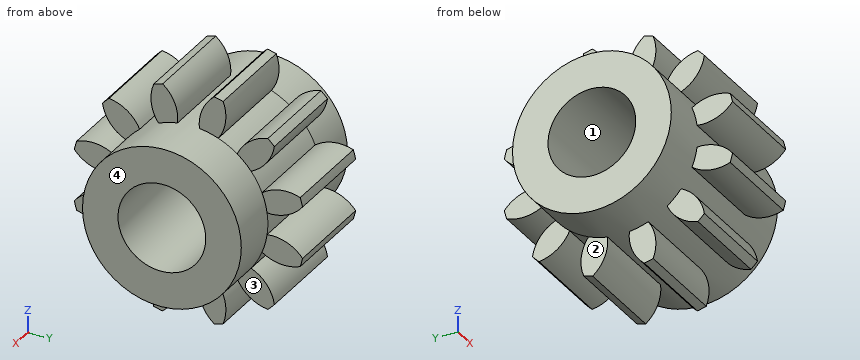
```python
from build123d import *
from build123d.topology import SkipClean

# Parameters (mm, degrees)
BASPROSKE_W       = 25.4
BASPROSKE_H       = 29.633333333
TOOTHCUT_DEPTH    = 50.004376222
TEETHCUTS_COUNT   = 12
TEETHCUTS_ANGLE   = 330
HUBNEABOTSKE_R    = 20.107063333
HUBNEARBOTH_DEPTH = 12.7000254
HUBFARSKE_R       = 20.107063333
HUBFAR_DEPTH      = 12.7000254
BORSKE_R          = 11.1125
BORE_DEPTH        = 50.8000508
SCALE1_SCALE      = 0.39


with BuildPart() as part:
    # BasProSke → Base-Revolve (revolve)
    with BuildSketch(Plane(origin=(0, 0, 0), x_dir=(1, 0, 0), z_dir=(0, 1, 0)), mode=Mode.PRIVATE) as base_revolve_sk:
        with Locations((12.7, 14.816666667)):
            Rectangle(BASPROSKE_W, BASPROSKE_H)
    revolve(base_revolve_sk.sketch.rotate(Axis((-10, 0, 0), (1, 0, 0)), 180), axis=Axis((-10, 0, 0), (1, 0, 0)))

    # TooCutSke → ToothCut (cut, through all)
    with BuildSketch(Plane(origin=(0, 0, 0), x_dir=(0, 0, -1), z_dir=(1, 0, 0))):
        with BuildLine():
            ThreePointArc((2.76285054, 19.91634135), (0, 20.107063333), (-2.76285054, 19.91634135))
            ThreePointArc((-2.76285054, 19.91634135), (-3.510108668, 24.907095847), (-6.566398379, 28.922705186))
            ThreePointArc((-6.566398379, 28.922705186), (0, 29.658733333), (6.566398379, 28.922705186))
            ThreePointArc((6.566398379, 28.922705186), (3.510108668, 24.907095847), (2.76285054, 19.91634135))
        make_face()
    toothcut = extrude(amount=TOOTHCUT_DEPTH, mode=Mode.SUBTRACT)

    # TeethCuts: ToothCut ×12 about axis
    teethcuts_axis = Axis((-10, 0, 0), (1, 0, 0))
    for i in range(1, TEETHCUTS_COUNT):
        add(toothcut.rotate(teethcuts_axis, i * TEETHCUTS_ANGLE / (TEETHCUTS_COUNT - 1)), mode=Mode.SUBTRACT)

    # HubNeaBotSke → HubNearBoth (add)
    with SkipClean():  # the faces are left unmerged after this step: merging them gives an invalid solid
        with BuildSketch(Plane.ZY):
            Circle(HUBNEABOTSKE_R)
        extrude(amount=HUBNEARBOTH_DEPTH)

    # HubFarSke → HubFar (add)
    with SkipClean():  # the faces are left unmerged after this step: merging them gives an invalid solid
        with BuildSketch(Plane(origin=(25.4, 0, 0), x_dir=(0, 0, -1), z_dir=(1, 0, 0))):
            with Locations(Location((0, 0, 0), (0, 0, 180))):
                Circle(HUBFARSKE_R)
        extrude(amount=HUBFAR_DEPTH)

    # BorSke → Bore (cut, symmetric)
    with SkipClean():  # the faces are left unmerged after this step: merging them gives an invalid solid
        with BuildSketch(Plane(origin=(0, 0, 0), x_dir=(0, 0, -1), z_dir=(1, 0, 0))):
            with Locations(Location((0, 0, 0), (0, 0, 180))):
                Circle(BORSKE_R)
        extrude(amount=BORE_DEPTH, both=True, mode=Mode.SUBTRACT)


with BuildPart() as part_1:
    # Scale1: scaled about (12.7, 0, 0)
    add(part.part.scale(SCALE1_SCALE).moved(Location((7.747, 0, 0))))


solid = part_1.part
```
CAD build for the part. Positions are in the model's coordinates, mm. Face numbers are marked on the shaded views. A direction names the side the tool comes from. Round coordinates to 2 decimals unless told otherwise and drop trailing zeros. Order: outer loops, then holes, each group sorted by start corner. A loop starts at its lowest first (then second) coordinate and runs counter-clockwise, first axis right, second up. Notation, with made-up numbers: (40, -26) -> (48, -26) arc R26 cw to (48, 5) -> close; hole circle Ø8 at (86, 40.25). An arc over 180 degrees is marked (long way). Write item = value, one per line.
(1) Cut at C-C (x = 6.75). Write the cut outline in (y, z).
Answers follow:
outline = circle Ø15.68 at (0, 0); hole circle Ø8.67 at (0, 0)
(2) Cut at B-B (y = -1.5). Write the cut outline in (x, z).
Answers follow:
outline = (2.79, -7.7) -> (7.75, -7.7) -> (7.75, -9.99) -> (17.65, -9.99) -> (17.65, -7.7) -> (22.61, -7.7) -> (22.61, -4.07) -> (2.79, -4.07) -> close; (2.79, 4.07) -> (22.61, 4.07) -> (22.61, 7.7) -> (17.65, 7.7) -> (17.65, 9.99) -> (7.75, 9.99) -> (7.75, 7.7) -> (2.79, 7.7) -> close
(3) Pull direction Y, two halves, no side cores. Call the marked faces 1 and 2: +Y half, -Y half, draft (parallel to the pull), parting line (faces both ways), or undercut.
Answers follow:
face_1 = undercut
face_2 = draft
(4) Flat gauge pins, fed straight in: P1, Ø1.3, axis at y = 9, z = 2, coming from the +X side; P2, Ø2, axis at y = 9.5, z = 2, coming from the -X side; P3, Ø3, axis at x = 14.5, z = -4.5, coming from the +Y side. Where does each tip first touch, or does it go through?
Answers follow:
P1 = 17.65
P2 = 7.75
P3 = 11.16
(5) Cut at A-A (z = 0). Write the cut outline in (x, y), plus the area to 3 significant figures.
Answers follow:
outline = (2.79, -7.84) -> (22.61, -7.84) -> (22.61, -4.33) -> (2.79, -4.33) -> close; (2.79, 4.33) -> (22.61, 4.33) -> (22.61, 7.84) -> (2.79, 7.84) -> close
area = 139 mm²
(6) Drill centre lines: L1, parallel to Y at x = 15, z = 0; L2, parallel to X at y = -2.25, z = 9; L3, parallel to Z at x = 16.75, y = -6.75. Where is each one in solid material? Low to high.
Answers follow:
L1 = -7.84 to -4.33, 4.33 to 7.84
L2 = 7.75 to 17.65
L3 = -8.16 to -5.13, -3.99 to 3.99, 5.13 to 8.16
(7) 3-axis set-ups, long thin cutter, end or side, ignore diameter. For the marked faces 3 and 4: which of +Z, -Z, +X, -X, +Y, -Y reach the whole face in a straight line?
Answers follow:
face_3 = -Z, +X, +Y
face_4 = +Z, -Z, +X, +Y, -Y
(8) Cut at D-D (y = -5.5). Write the cut outline in (x, z), plus the area to 3 significant figures.
Answers follow:
outline = (2.79, -5.59) -> (7.75, -5.59) -> (7.75, -7.23) -> (17.65, -7.23) -> (17.65, -5.59) -> (22.61, -5.59) -> (22.61, 5.59) -> (17.65, 5.59) -> (17.65, 7.23) -> (7.75, 7.23) -> (7.75, 5.59) -> (2.79, 5.59) -> close
area = 254 mm²
